Work out the finished part from the listing and answer in its coordinate system (mm). Face numbers are marked on the shaded views. A direction names the side the tool comes from. Coordinates: 2 decimals unless noted, no trailing zeros. Order: outer loops, then holes, each group sorted by start corner. A loop starts at its lowest first (then second) coordinate and runs counter-clockwise, first axis right, second up.
Autodesk Inventor part; units mm, degrees
ref_plane "YZ Plane" through (0, 0, 0) normal (1, 0, 0) x (0, 1, 0)
ref_plane "XZ Plane" through (0, 0, 0) normal (0, 1, 0) x (-1, 0, 0)
ref_plane "XY Plane" through (0, 0, 0) normal (0, 0, 1) x (1, 0, 0)
sketch "Sketch1" plane through (0, 0, 0) normal (0, 0, 1) x (1, 0, 0)
  circle A0 centre (11.9875, 17.6045) radius 7.5
  arc A1 (18.7629, 10.9455) -> (7.7868, 26.1253) centre (11.9875, 17.6045) ccw
  line L0 (-8.0125, -7.3955) -> (-0.0125, -7.3955) construction
  line L1 (-0.0125, -7.3955) -> (-0.0125, 4.8295) construction
  line L2 (16.9875, 9.139) -> (16.9875, -32.861)
  line L3 (16.9875, -32.861) -> (-23.0125, -32.861)
  line L4 (-23.0125, -32.861) -> (-23.0125, 10.9414)
  line L5 (37.2097, -0.3955) -> (-34.0078, -0.3955) construction
  line L6 (31.0948, -7.8955) -> (-30.4036, -7.8955) construction
  line L7 (29.7312, 7.1045) -> (-30.4036, 7.1045) construction
  line L8 (-23.0125, 10.9414) -> (7.7868, 26.1253)
  line L9 (16.9875, 9.139) -> (18.7629, 10.9455)
  dimension "d1" = 2
  dimension "d2" = 15
  dimension "d3" = 25
  dimension "d4" = 20
  dimension "d5" = 8
  dimension "d6" = 42
  dimension "d7" = 5
  dimension "d8" = 18
  dimension "d10" = 15
  dimension "d11" = 15
  dimension "d12" = 40
extrude "Extrusion1" add sketch "Sketch1" along normal blind 25
sketch "Sketch2" plane through (-23.0125, -32.861, 0) normal (-1, 0, 0) x (0, 0, 1)
  line L0 (0, 43.8024) -> (0, 0) construction
  line L1 (25, 57.9655) -> (25, 42.9655) construction
  line L2 (0, 42.9655) -> (0, 57.9655) construction
  line L3 (25, 50.4655) -> (0, 50.4655) construction
  line L4 (25, 57.9655) -> (0, 57.9655) construction
  line L5 (25, 42.9655) -> (0, 42.9655) construction
  line L6 (25, 57.9655) -> (25, 42.9655) construction
  line L7 (37.5603, 32.4655) -> (-20.7807, 32.4655) construction
  circle A0 centre (9.5, 32.4655) radius 7.5
  point P0 (0, 32.861)
  dimension "d15" = 15
  dimension "d16" = 15
  dimension "d17" = 15
  dimension "d19" = 18
  dimension "d20" = 9.5
extrude "Y Glide hul" cut sketch "Sketch2" against normal up to surface (40 mm away)
sketch "Sketch25" plane through (0, 0, 25) normal (0, 0, 1) x (1, 0, 0)
  line L0 (-23.0125, -32.861) -> (16.9875, -32.861)
  line L1 (-23.0125, 10.9414) -> (-23.0125, -32.861)
  line L2 (16.9875, -32.861) -> (-23.0125, -32.861)
  line L3 (-23.0125, -32.861) -> (-23.0125, -10.861)
  line L4 (-23.0125, -10.861) -> (16.9875, -10.861)
  line L5 (16.9875, -10.861) -> (16.9875, -32.861)
  dimension "d150" = 22
extrude "Extrusion23" cut sketch "Sketch25" against normal blind 20
ref_plane "Work Plane7" through (-0.0125, -32.861, 0) normal (-1, 0, 0) x (0, 0, 1)
sketch "Sketch29" plane through (-0.0125, -32.861, 0) normal (-1, 0, 0) x (0, 0, 1)
  line L0 (5, 22) -> (25, 22) construction
  line L1 (25, 43.8024) -> (25, 22) construction
  line L2 (0, 43.8024) -> (25, 43.8024) construction
  line L3 (0, 43.8024) -> (0, 0) construction
  line L4 (0, 0) -> (5, 0) construction
  line L5 (5, 0) -> (5, 22) construction
  circle A0 centre (9.5, 32.4655) radius 7.5 construction
  line L6 (5, 22) -> (5, 0)
  line L7 (5, 0) -> (5, 10)
  line L8 (5, 10) -> (15, 10)
  line L9 (15, 10) -> (15, 16)
  line L10 (15, 16) -> (5, 16)
  line L11 (21, 3) -> (21, 19.5032) construction
  point P0 (0, 32.861)
  dimension "d154" = 10
  dimension "d155" = 10
  dimension "d156" = 6
  dimension "d170" = 6
revolve "Revolution2" add sketch "Sketch29" angle 180 mid plane about axis through (-0.0125, -29.861, 21) along (0, 1, 0)
sketch "Sketch30" plane through (5.9875, -22.861, 21) normal (0, -1, 0) x (1, 0, 0)
  line L0 (10, 0) -> (0, 0)
  arc A0 (-12, 0) -> (0, 0) centre (-6, 0) ccw
  line L1 (-22, 0) -> (-12, 0)
  arc A1 (-22, 0) -> (-6, -16) centre (-6, 0) ccw
  arc A2 (-6, -16) -> (10, 0) centre (-6, 0) ccw
  arc A3 (-12, 0) -> (0, 0) centre (-6, 0) ccw
  line L2 (10, 0) -> (0, 0)
  line L3 (10, 0) -> (0, 0)
  line L4 (-12, 0) -> (-22, 0)
  line L5 (11, -16) -> (-29, -16)
  line L6 (-29, -21) -> (-29, -16)
  line L7 (-29, -21) -> (11, -21)
  line L8 (11, -21) -> (11, -16)
  line L9 (-22, 0) -> (-22, -16)
  line L10 (-22, -16) -> (-6, -16)
  line L11 (10, 0) -> (10, -16)
  line L12 (10, -16) -> (-6, -16)
  point P0 (-5.9875, -21)
extrude "Extrusion24" add sketch "Sketch30" against normal up to surface (6 mm away) contours A2 A1 L1 A0 L0 | L11 L5 A2 | L5 L9 A1
sketch "Sketch32" plane through (-0.0125, -22.861, 21) normal (0, -1, 0) x (1, 0, 0)
  line L0 (16, 0) -> (6, 0)
  arc A0 (-6, 0) -> (6, 0) centre (0, 0) ccw
  line L1 (-16, 0) -> (-6, 0)
  line L2 (-16, 0) -> (-16, -16)
  line L3 (16, -16) -> (-16, -16)
  line L4 (16, -16) -> (16, 0)
  line L5 (16, -16) -> (16, 0)
  line L6 (16, 0) -> (16, -16)
  line L7 (16, -16) -> (-3, -16)
  line L8 (-23, -16) -> (17, -16)
  line L9 (-16, 0) -> (-16, -16)
  line L10 (-3, -16) -> (-16, -16)
  line L11 (-16, -16) -> (-16, 0)
  arc A1 (-8, 0) -> (8, 0) centre (0, 0) ccw
  line L12 (6, 0) -> (16, 0)
  line L13 (16, -16) -> (16, 0)
  line L14 (-16, -16) -> (16, -16)
  line L15 (-16, 0) -> (-16, -16)
  line L16 (-6, 0) -> (-16, 0)
  arc A2 (-6, 0) -> (6, 0) centre (0, 0) ccw
  point P0 (0.0125, -21)
  dimension "d171" = 16
extrude "Extrusion25" add sketch "Sketch32" along normal up to surface (10 mm away) contours L4 L3 L2 L1 A1 L0
sketch "Sketch35" plane through (15.9875, -32.861, 5) normal (1, 0, 0) x (0, 0, -1)
  line L0 (0, 16) -> (-16, 16)
  line L1 (-16, 16) -> (-16, 0)
  line L2 (-16, 0) -> (0, 0)
  line L3 (0, 16) -> (0, 0)
  line L4 (-13, 7) -> (-13, 0)
  line L5 (-13, 0) -> (0, 0)
  line L6 (0, 0) -> (0, 16)
  line L7 (0, 16) -> (-13, 16)
  line L8 (-13, 16) -> (-13, 0)
  point P0 (5, 32.861)
extrude "Extrusion26" add sketch "Sketch35" along normal up to surface (1 mm away) contours L3 L2 L4 L8 L0
sketch "Sketch36" plane through (-16.0125, -32.861, 5) normal (-1, 0, 0) x (0, 0, 1)
  line L0 (16, 16) -> (0, 16)
  line L1 (0, 0) -> (0, 16)
  line L2 (0, 0) -> (16, 0)
  line L3 (16, 16) -> (16, 0)
  line L4 (16, 10) -> (16, 16)
  line L5 (16, 16) -> (0, 16)
  line L6 (0, 16) -> (0, 0)
  line L7 (0, 0) -> (16, 0)
  line L8 (16, 0) -> (16, 16)
  point P0 (-5, 32.861)
extrude "Extrusion27" add sketch "Sketch36" along normal up to surface (7 mm away)
sketch "Sketch38" plane through (-23.0125, -32.861, 0) normal (-1, 0, 0) x (0, 0, 1)
  line L0 (5, 22) -> (25, 22)
  line L1 (25, 43.8024) -> (25, 22)
  line L2 (0, 43.8024) -> (25, 43.8024)
  line L3 (0, 43.8024) -> (0, 0)
  line L4 (0, 0) -> (21, 0)
  line L5 (21, 16) -> (21, 0)
  line L6 (5, 16) -> (21, 16)
  line L7 (5, 16) -> (5, 22)
  circle A0 centre (9.5, 32.4655) radius 7.5
  line L8 (0, 43.8024) -> (25, 43.8024)
  line L9 (0, 43.8024) -> (0, 64.0171)
  line L10 (0, 64.0171) -> (25, 64.0171)
  line L11 (25, 64.0171) -> (25, 43.8024)
  line L12 (5, 43.8024) -> (0, 43.8024)
  line L13 (25, 43.8024) -> (0, 43.8024)
  point P0 (0, 32.861)
extrude "Extrusion28" cut sketch "Sketch38" against normal blind 13
ref_plane "Work Plane8" through (-0.0125, -16.861, 21) normal (0, 1, 0) x (1, 0, 0)
sketch "Sketch39" plane through (-0.0125, -16.861, 21) normal (0, 1, 0) x (1, 0, 0)
  arc A0 (8, 0) -> (-8, 0) centre (0, 0) ccw
  line L0 (8, 0) -> (6, 0)
  arc A1 (6, 0) -> (-6, 0) centre (0, 0) ccw
  line L1 (-8, 0) -> (-6, 0)
  circle A2 centre (0, 0) radius 3
  point P0 (0.0125, 21)
  dimension "d173" = 6
extrude "Bowden slange hul" cut sketch "Sketch39" along normal blind 56 contours A2
sketch "Sketch40" plane through (7.9875, -32.861, 21) normal (0, -1, 0) x (1, 0, 0)
  line L0 (-18, 0) -> (-18, -21)
  line L1 (-18, -21) -> (9, -21)
  line L2 (9, -21) -> (9, -3)
  line L3 (8, -3) -> (9, -3)
  line L4 (8, 0) -> (8, -3)
  line L5 (0, 0) -> (8, 0)
  arc A0 (-16, 0) -> (0, 0) centre (-8, 0) ccw
  line L6 (-18, 0) -> (-16, 0)
  point P0 (-7.9875, -21)
extrude "Extrusion30" cut sketch "Sketch40" against normal blind 4
sketch "Sketch41" plane through (15.9875, -16.861, 18) normal (0, 0, 1) x (1, 0, 0)
  line L0 (0, -12) -> (1, -12)
  line L1 (1, -12) -> (1, 0)
  line L2 (0, 0) -> (1, 0)
  line L3 (0, -12) -> (0, 0)
  point P0 (-15.9875, 16.861)
extrude "Extrusion31" add sketch "Sketch41" along normal up to surface (3 mm away)
sketch "Sketch42" plane through (5.9875, -16.861, 21) normal (0, 0, 1) x (1, 0, 0)
  circle A0 centre (5, -6) radius 2
  line L0 (0, 0) -> (11, 0)
  line L1 (11, 0) -> (11, -12)
  point P0 (-5.9875, 16.861)
  dimension "d180" = 4
  dimension "d181" = 6
  dimension "d182" = 6
extrude "Holder montering" cut sketch "Sketch42" against normal up to surface (21 mm away)
sketch "Sketch43" plane through (-10.0125, -32.861, 0) normal (-1, 0, 0) x (0, 0, 1)
  circle A0 centre (9.5, 32.4655) radius 7.5
  line L0 (0, 4) -> (21, 4)
  line L1 (21, 16) -> (21, 4)
  line L2 (5, 16) -> (21, 16)
  line L3 (5, 22) -> (5, 16)
  line L4 (25, 22) -> (5, 22)
  line L5 (25, 50.2113) -> (25, 22)
  line L6 (0, 50.2113) -> (25, 50.2113) construction
  line L7 (0, 4) -> (0, 50.2113)
  line L8 (25, 50.2113) -> (25, 62.2894)
  line L9 (25, 62.2894) -> (0, 62.2894)
  line L10 (0, 50.2113) -> (25, 50.2113) construction
  line L11 (0, 62.2894) -> (0, 50.2113)
  point P0 (0, 32.861)
extrude "Extrusion33" cut sketch "Sketch43" against normal blind 3
equation "\"d11\" = d10"
equation "\"d16\" = d15"
properties part number "Main" material "PLA Plastic"
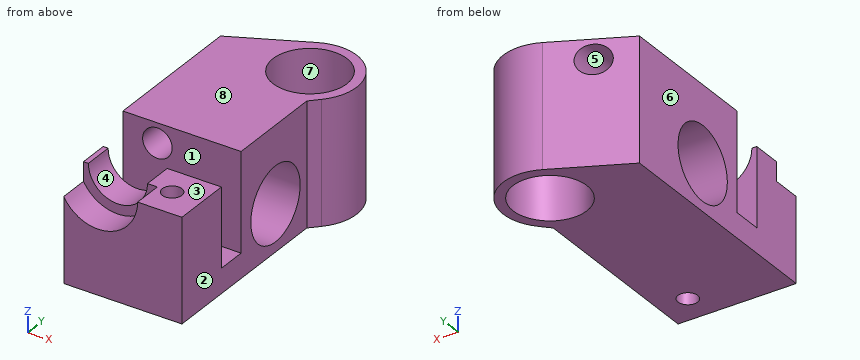
1. For the marked faces 1, 2, 3 and 4, determine the directions among +Z, -Z, +X, -X, +Y, -Y from which every point of the face is accessible in a straight line to the end or side of a thin tool.
2. The part is cut by section B-B (z = 5.75). Determine the outline of the cut face in (x, y), plus the area to 3 significant figures.
3. Flat-ended cylindrical pins translate along their axes: pin 1 (0.5 mm diameter, centred on x = -6.5, y = -19, fed in from +Z); pin 2 (5 mm diameter, centred on x = 1.5, y = -15, fed in from +Z); pin 3 (13 mm diameter, centred on x = 1.5, z = 15, fed in from +Y). Find the tip coordinate at first contact, or state that the pin passes through.
4. The part is cut by section D-D (x = 11.5). Determine the outline of the cut face in (y, z).
5. The part is cut by section A-A (x = 0.75). Determine the outline of the cut face in (y, z).
6. The part is cut by section C-C (y = 3.5). Determine the outline of the cut face in (x, z).
7. Consider probe 1 along X at (y, z) = (9, 21); probe 2 along X at (y, z) = (17.5, 16.5); probe 3 along Y at (x, z) = (16, 12). Determine where each line is inside the solid, lowest interval first.
8. The mould has two halves that part along X. Classify the marked faces 5, 6, 7 and 8: released by +X, released by -X, zero draft, split by the parting line, or undercut.
Worked out:
1. face 1: +Z, +X, -X
1. face 2: +Z, -Z, +X, -Y
1. face 3: +Z, +X, -X, -Y
1. face 4: +Z, -Y
2. outline: (-7.01, -28.86) - (16.99, -28.86) - (16.99, -16.86) - (-7.01, -16.86) - close; (-7.01, -10.86) - (16.99, -10.86) - (16.99, -6.89) - (-7.01, -6.89) - close; (-7.01, 6.1) - (16.99, 6.1) - (16.99, 9.14) - (18.76, 10.95) arc R9.5 ccw to (7.79, 26.13) - (-7.01, 18.83) - close; hole circle Ø15 at (11.99, 17.6); hole circle Ø4 at (10.99, -22.86)
2. area: 678 mm2
3. pin 1: stops at z = 21
3. pin 2: stops at z = 15.91
3. pin 3: stops at y = 26.23
4. outline: (-28.86, 0) - (-24.79, 0) - (-24.79, 21) - (-28.86, 21) - close; (-20.93, 0) - (10.12, 0) - (10.12, 25) - (-10.86, 25) - (-10.86, 5) - (-16.86, 5) - (-16.86, 21) - (-20.93, 21) - close; (25.09, 0) - (27.09, 0) - (27.09, 25) - (25.09, 25) - close; hole circle Ø15 at (-0.4, 9.5)
5. outline: (-28.86, 0) - (22.66, 0) - (22.66, 18.1) - (-10.86, 18.1) - (-10.86, 5) - (-16.86, 5) - (-16.86, 15.05) - (-22.86, 15.05) - (-22.86, 13.04) - (-28.86, 13.04) - close; (-10.86, 23.9) - (22.66, 23.9) - (22.66, 25) - (-10.86, 25) - close; hole circle Ø15 at (-0.4, 9.5)
6. outline: (-7.01, 0) - (16.99, 0) - (16.99, 3.09) - (-7.01, 3.09) - close; (-7.01, 15.91) - (16.99, 15.91) - (16.99, 25) - (-7.01, 25) - close; hole circle Ø6 at (-0.01, 21)
7. probe 1: x = -7.01 to -3.01, 2.99 to 16.99
7. probe 2: x = -7.01 to 4.49, 19.49 to 21.49
7. probe 3: y = -28.86 to -16.86, -10.86 to -7.47, 6.68 to 11.27, 23.94 to 26.22
8. face 5: undercut
8. face 6: released by -X
8. face 7: undercut
8. face 8: zero draft
